Here's how the part is built. I have some questions about the finished solid (model axes, mm). Round coordinates to 2 decimals unless told otherwise and drop trailing zeros. Write each loop counter-clockwise with the first axis right and the second up, starting at its lowest first coordinate (ties: lowest second). Pieces come first, ordered by that corner, then holes. Notation, with made-up numbers: (-2, -18.75) -> (55, -18.75) arc R28 ccw to (55, -0.75) -> close; hole circle Ø5 at (45.5, -1). An arc over 180 degrees is marked (long way). Put each result on its own line as item: value. Start each with the question number.
1. For pin 1 (5.5 mm diameter, centred on x = 0, z = -50.8, fed in from -Y) (3 decimals); pin 2 (1.5 mm diameter, centred on y = 2, z = -97.5, fed in from +X) (3 decimals), each with a flat end and sliding along its axis, tell me the tip position at first contact or that it passes through.
2. Suppose I cut it at C-C (y = 1.65). Please give me the cut outline in (x, z) (3 decimals), then the cut area to 3 significant figures.
3. I need wall thicknesses on probe 1 along Z at (x, y) = (0, 2) (3 decimals); probe 2 along X at (y, z) = (2.9, -10.5); probe 3 along Z at (x, y) = (101.6, 2.1) (3 decimals). Which ranges of each line are inside material? Lowest first, please. Write a range as from..to.
4. Suppose I cut it at A-A (x = 0). Please give me the cut outline in (y, z) (3 decimals), then the cut area to 3 significant figures.
5. Suppose I cut it at D-D (z = -12.7). Please give me the cut outline in (x, y) (3 decimals), then the cut area to 3 significant figures.
6. We'd pull the mould along X, two halves only. Please class faces 1 (the face through (2, 3.175, -60)), 2 (the face through (69.05, 1.57, -89.79)), 3 (the face through (-0.41, 1.57, -53.95)): +X half, -X half, draft (parallel to the pull), parting line (faces both ways), or undercut.
7. Suppose I cut it at B-B (z = -50.8). Please give me the cut outline in (x, y) (3 decimals), then the cut area to 3 significant figures.
```python
from build123d import *

# Parameters (mm, degrees)
SKETCH1_R           = 3.175
BOSS_EXTRUDE1_DEPTH = 3.175


with BuildPart() as part:
    # Sketch1 → Boss-Extrude1 (new body)
    with BuildSketch(Plane(origin=(0, 0, 0), x_dir=(1, 0, 0), z_dir=(0, 1, 0))):
        Polygon((127, 0), (-127, 0), (-127, 25.4), (-12.7, 152.4), (12.7, 152.4), (127, 25.4), align=None)
        with Locations((0, 127)):
            Circle(SKETCH1_R, mode=Mode.SUBTRACT)
        with Locations((0, 50.8)):
            Circle(SKETCH1_R, mode=Mode.SUBTRACT)
        with Locations((-101.6, 12.7)):
            Circle(SKETCH1_R, mode=Mode.SUBTRACT)
        with Locations((101.6, 12.7)):
            Circle(SKETCH1_R, mode=Mode.SUBTRACT)
    extrude(amount=BOSS_EXTRUDE1_DEPTH)


solid = part.part
```
Verdict:
1. pin 1: passes through
1. pin 2: stops at x = 62.785
2. outline: (-127, -25.4) -> (-12.7, -152.4) -> (12.7, -152.4) -> (127, -25.4) -> (127, 0) -> (-127, 0) -> close; hole circle Ø6.35 at (-101.6, -12.7); hole circle Ø6.35 at (0, -127); hole circle Ø6.35 at (0, -50.8); hole circle Ø6.35 at (101.6, -12.7)
2. area: 24,100 mm^2
3. probe 1: z = -152.4..-130.175, -123.825..-53.975, -47.625..0
3. probe 2: x = -127..-103.89, -99.31..99.31, 103.89..127
3. probe 3: z = -53.622..-15.875, -9.525..0
4. outline: (0, -152.4) -> (3.175, -152.4) -> (3.175, -130.175) -> (0, -130.175) -> close; (0, -123.825) -> (3.175, -123.825) -> (3.175, -53.975) -> (0, -53.975) -> close; (0, -47.625) -> (3.175, -47.625) -> (3.175, 0) -> (0, 0) -> close
4. area: 444 mm^2
5. outline: (-127, 0) -> (-104.775, 0) -> (-104.775, 3.175) -> (-127, 3.175) -> close; (-98.425, 0) -> (98.425, 0) -> (98.425, 3.175) -> (-98.425, 3.175) -> close; (104.775, 0) -> (127, 0) -> (127, 3.175) -> (104.775, 3.175) -> close
5. area: 766 mm^2
6. face 1: draft
6. face 2: +X half
6. face 3: undercut
7. outline: (-104.14, 0) -> (-3.175, 0) -> (-3.175, 3.175) -> (-104.14, 3.175) -> close; (3.175, 0) -> (104.14, 0) -> (104.14, 3.175) -> (3.175, 3.175) -> close
7. area: 641 mm^2
